```python
from build123d import *

# Parameters (mm, degrees)
BOSS_EXTRUDE1_DEPTH = 3
SKETCH2_W           = 3
SKETCH2_H           = 250.046113764
BOSS_EXTRUDE2_DEPTH = 6.35
CHAMFER1_SIZE       = 1.3
CHAMFER2_SIZE       = 1.3
CHAMFER3_SIZE       = 1.3


with BuildPart() as part:
    # Sketch1 → Boss-Extrude1 (new body)
    with BuildSketch(Plane.XY):
        Polygon((60, 2660), (59.981247069, 2660), (59.981247069, 2359.953886236), (182, 2660), (182, 2716), align=None)
    extrude(amount=BOSS_EXTRUDE1_DEPTH)

    # Sketch2 → Boss-Extrude2 (add)
    with BuildSketch(Plane.ZY.offset(-59.981247069)):
        with Locations((1.5, 2534.976943118)):
            Rectangle(SKETCH2_W, SKETCH2_H)
    extrude(amount=BOSS_EXTRUDE2_DEPTH)

    # Chamfer1
    chamfer1_edges = [part.edges().sort_by_distance(p)[0] for p in [
        (120.990623535, 2509.976943118, 3),
        (120.990623535, 2509.976943118, 0),
    ]]
    chamfer(chamfer1_edges, length=CHAMFER1_SIZE)

    # Chamfer2
    chamfer2_edges = [part.edges().sort_by_distance(p)[0] for p in [
        (121, 2688, 3),
        (121, 2688, 0),
    ]]
    chamfer(chamfer2_edges, length=CHAMFER2_SIZE)

    # Chamfer3
    chamfer3_edges = [part.edges().sort_by_distance(p)[0] for p in [
        (182, 2689.010267295, 0),
        (182, 2689.010267295, 3),
    ]]
    chamfer(chamfer3_edges, length=CHAMFER3_SIZE)


solid = part.part
```
The model under review builds one solid part; all positions refer to its coordinate system, in mm. Round coordinates to 2 decimals unless told otherwise and drop trailing zeros. Loops run counter-clockwise (first coordinate to the right, second up) from the corner with the lowest first, then second, coordinate; pieces in that order, holes last.
Item 1: Take a section at B-B (x = 132). Write out the cut boundary in (y, z).
Determined:
outline: (2537.05, 1.3) - (2540.5, 0) - (2691.62, 0) - (2693.05, 1.3) - (2693.05, 1.7) - (2691.62, 3) - (2540.5, 3) - (2537.05, 1.7) - close
Item 2: Take a section at C-C (y = 2473.5). Write out the cut boundary in (x, z).
Determined:
outline: (53.63, 0) - (104.75, 0) - (106.16, 1.3) - (106.16, 1.7) - (104.75, 3) - (53.63, 3) - close
Item 3: Take a section at A-A (z = 0.65). Write out the cut boundary in (x, y), then the cut area to 3 significant figures.
Determined:
outline: (53.63, 2409.95) - (59.98, 2409.95) - (59.98, 2361.68) - (181.35, 2660.13) - (181.35, 2714.99) - (61.56, 2660) - (53.63, 2660) - close
area: 23,000 mm2
Item 4: Take a section at D-D (x = 163). Write out the cut boundary in (y, z), then the cut area to 3 significant figures.
Determined:
outline: (2613.28, 1.3) - (2616.73, 0) - (2705.85, 0) - (2707.28, 1.3) - (2707.28, 1.7) - (2705.85, 3) - (2616.73, 3) - (2613.28, 1.7) - close
area: 276 mm2
Item 5: For line 1 (X direction, y = 2573, z = 0.3); line 2 (X direction, y = 2399, z = 1.25); line 3 (Y direction, x = 102, z = 1.5), list the stretches that pass through material, from the lowest coordinate up.
Determined:
line 1: x = 53.63 to 145.54
line 2: x = 59.98 to 75.81
line 3: y = 2463.28 to 2679.28
Item 6: Clearance check with flat-ended pins moving along their axes: pin 1 Ø1.5 at (y, z) = (2389.5, 1.5) entering from -X; pin 2 Ø1.5 at (y, z) = (2456.5, 1.5) entering from +X. State where each tip first meets the part, or that it passes through.
Determined:
pin 1: stops at x = 59.98
pin 2: stops at x = 99.55
